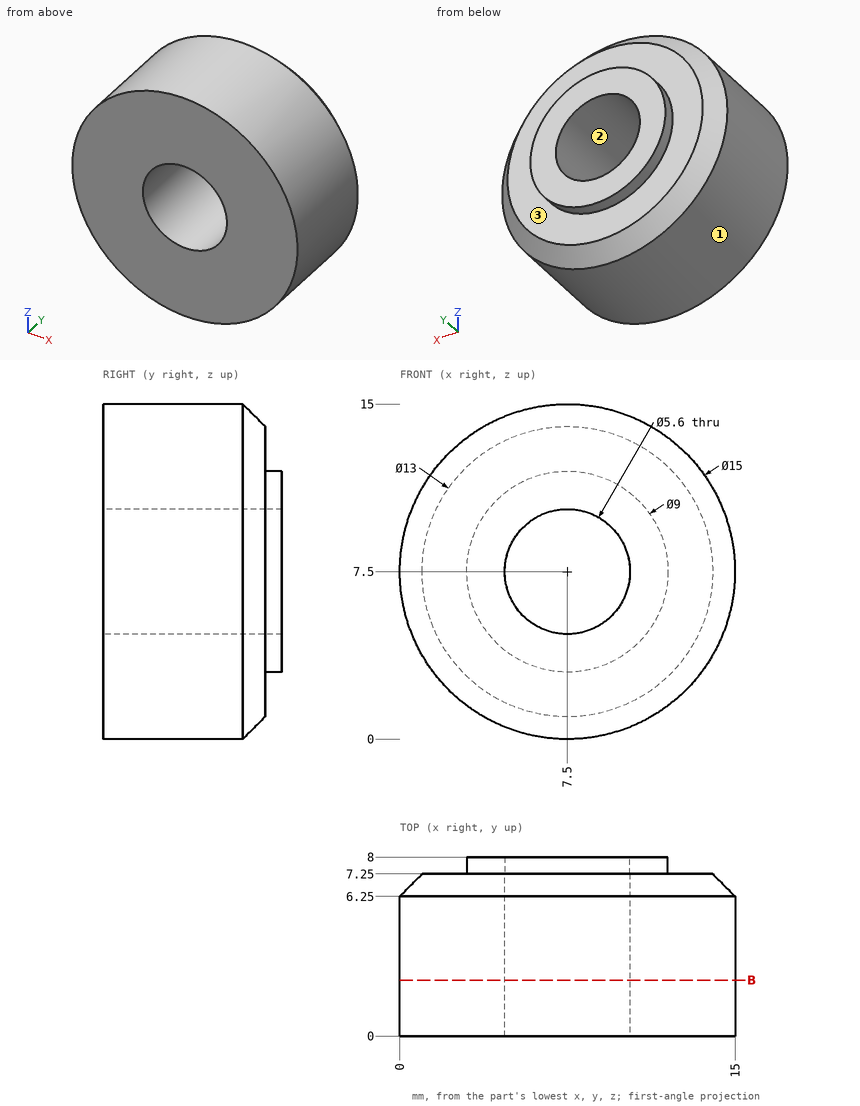
Verification items for this drawing (mm, ordinates from the low corner). Coordinates: 2 decimals unless noted, no trailing zeros. Loops run counter-clockwise (first coordinate to the right, second up) from the corner with the lowest first, then second, coordinate; pieces in that order, holes last. Notation, with made-up numbers: (38.25, 75.25) -> (46.25, 75.25) arc R26 ccw to (46.25, 97.25) -> close; hole circle Ø8 at (-39.5, -29). An arc over 180 degrees is marked (long way). Put each result on its own line as item: value.
1. Mould release check, pull along Z, two halves, no side actions. Record for the marked faces 1, 2 and 3: pulls with the +Z half, pulls with the -Z half, needs draft (parallel to the pull), parting line crosses it, or undercut.
Result set:
face 1: parting line crosses it
face 2: undercut
face 3: needs draft
2. Gauge pin test, flat ends, axial feed: P1, Ø3, axis at x = 4.5, y = 2.5, coming from the +Z side; P2, Ø4, axis at y = 7, z = 8.5, coming from the +X side. Record the tip position at first contact, or that the pin passes through.
Result set:
P1: stops at z = 14.85
P2: stops at x = 15
3. Section check B-B, the plane y = 2.5. Record the boundary of the cut face in (x, z), then the cut area to 3 significant figures.
Result set:
outline: circle Ø15 at (7.5, 7.5); hole circle Ø5.6 at (7.5, 7.5)
area: 152 mm^2
4. Thickness scan on line 1 (Z direction, x = 7.5, y = 4.25); line 2 (Y direction, x = 11.25, z = 3.75); line 3 (Z direction, x = 5, y = 3.75). Record the ranges inside material, lowest first.
Result set:
line 1: z = 0 to 4.7, 10.3 to 15
line 2: y = 0 to 7.25
line 3: z = 0.43 to 6.24, 8.76 to 14.57
